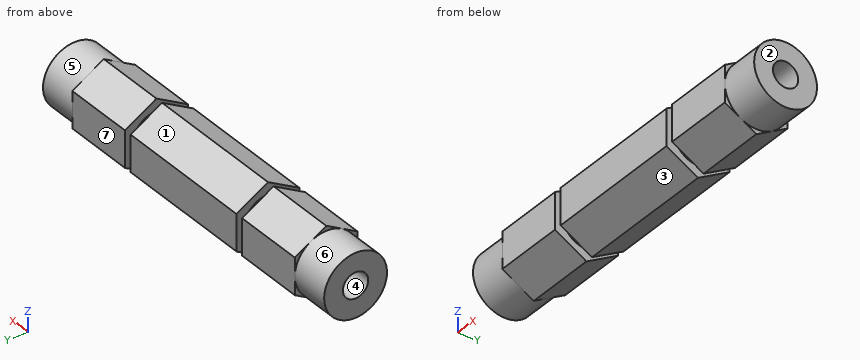
Autodesk Inventor part; units mm, degrees
ref_plane "YZ Plane" through (0, 0, 0) normal (1, 0, 0) x (0, 1, 0)
ref_plane "XZ Plane" through (0, 0, 0) normal (0, 1, 0) x (-1, 0, 0)
ref_plane "XY Plane" through (0, 0, 0) normal (0, 0, 1) x (1, 0, 0)
sketch "Sketch1" plane through (0, 0, 0) normal (1, 0, 0) x (0, 1, 0)
  line L0 (0, -7.3323) -> (-6.35, -3.6662)
  line L1 (-6.35, -3.6662) -> (-6.35, 3.6662)
  line L2 (-6.35, 3.6662) -> (0, 7.3323)
  line L3 (0, 7.3323) -> (6.35, 3.6662)
  line L4 (6.35, 3.6662) -> (6.35, -3.6662)
  line L5 (6.35, -3.6662) -> (0, -7.3323)
  point P0 (0, 0)
  point P1 (0, 0)
  dimension "d0" = 12.7
extrude "Extrusion1" add sketch "Sketch1" along normal mid plane 60.2996
sketch "Sketch2" plane through (-30.1498, 0, 0) normal (-1, 0, 0) x (0, 0, 1)
  circle A0 centre (0, 0) radius 6.35
  dimension "d3" = 12.7
extrude "Extrusion2" add sketch "Sketch2" along normal blind 7.9502
sketch "Sketch3" plane through (30.1498, 0, 0) normal (1, 0, 0) x (0, 0, -1)
  circle A0 centre (0, 0) radius 6.35
  line L0 (3.6662, 6.35) -> (-3.6662, 6.35)
  line L1 (-3.6662, 6.35) -> (-7.3323, 0)
  line L2 (-7.3323, 0) -> (-3.6662, -6.35)
  line L3 (-3.6662, -6.35) -> (3.6662, -6.35)
  line L4 (3.6662, -6.35) -> (7.3323, 0)
  line L5 (7.3323, 0) -> (3.6662, 6.35)
  dimension "d6" = 12.7
extrude "Extrusion3" add sketch "Sketch3" along normal blind 7.9502 contours A0
sketch "Sketch4" plane through (38.1, 0, 0) normal (1, 0, 0) x (0, 0, -1)
  point P0 (0, 0)
  point P1 (0, 0)
hole "Hole1" at (38.1, 0, 0) direction (-1, 0, 0) diameter 5.1054 end through all
sketch "Sketch6" plane through (0, 0, 0) normal (0, 1, 0) x (-1, 0, 0)
  line L0 (30.1498, 6.35) -> (38.1, 6.35)
  line L1 (38.1, 6.35) -> (38.1, 2.5527)
  line L2 (38.1, 2.5527) -> (-38.1, 2.5527)
  line L3 (-38.1, 2.5527) -> (-38.1, 6.35)
  line L4 (-38.1, 6.35) -> (-30.1498, 6.35)
  line L5 (-30.1498, 6.35) -> (-30.1498, 7.3323)
  line L6 (-30.1498, 7.3323) -> (30.1498, 7.3323)
  line L7 (30.1498, 7.3323) -> (30.1498, 6.35)
  line L8 (38.1, -6.35) -> (30.1498, -6.35)
  line L9 (30.1498, -6.35) -> (30.1498, -7.3323)
  line L10 (30.1498, -7.3323) -> (-30.1498, -7.3323)
  line L11 (-30.1498, -7.3323) -> (-30.1498, -6.35)
  line L12 (-30.1498, -6.35) -> (-38.1, -6.35)
  line L13 (-38.1, -6.35) -> (-38.1, -2.5527)
  line L14 (-38.1, -2.5527) -> (38.1, -2.5527)
  line L15 (38.1, -2.5527) -> (38.1, -6.35)
  line L16 (38.1, 2.5527) -> (38.1, -2.5527)
  line L17 (38.1, 0) -> (-38.1, 0)
  line L18 (-38.1, 6.35) -> (-38.1, -6.35)
  line L19 (15.875, -7.3323) -> (14.351, -7.3323)
  line L20 (14.351, -7.3323) -> (14.351, -4.9784)
  line L21 (14.351, -4.9784) -> (15.875, -4.9784)
  line L22 (15.875, -4.9784) -> (15.875, -7.3323)
  point P0 (0, 0)
  dimension "d16" = 9.9568
  dimension "d17" = 1.524
  dimension "d18" = 22.225
revolve "Revolution1" cut sketch "Sketch6" angle 360 about axis through (-38.1, 0, 0) along (1, 0, 0) contours L10 L20 L21 L22
mirror "Mirror1" about plane through (0, 0, 0) normal (1, 0, 0) of "Revolution1"
properties part number "EL2-GB-005E-grove" material "Aluminum 6061"
Design review of the part built by this model. Coordinates are the model's own, in mm. Face numbers are marked on the shaded views. A direction names the side the tool comes from. Give positions to 0.01 mm unless a question says otherwise; leave off trailing zeros. Write each loop counter-clockwise with the first axis right and the second up, starting at its lowest first coordinate (ties: lowest second). Pieces come first, ordered by that corner, then holes. Notation, with made-up numbers: (27, 86) -> (31, 86) arc R15 ccw to (31, 110) -> close; hole circle Ø10 at (-23, -13). An arc over 180 degrees is marked (long way). Answer in a Markdown table with one row per item.
(1) To check wall thickness, follow probe 1 along X at (y, z) = (3.5, 4) (3 decimals); probe 2 along X at (y, z) = (0.25, 6.5) (3 decimals); probe 3 along Y at (x, z) = (13, 0.25). State the ranges of each line that lie inside material, in increasing order.
Results:
| item | result |
|---|---|
| probe 1 | -38.1 to -15.875, -14.351 to 14.351, 15.875 to 38.1 |
| probe 2 | -30.15 to -15.875, -14.351 to 14.351, 15.875 to 30.15 |
| probe 3 | -6.35 to -2.54, 2.54 to 6.35 |
(2) Clearance check with flat-ended pins moving along their axes: pin 1 (4.5 mm diameter, centred on y = 0, z = 0, fed in from -X); pin 2 (1 mm diameter, centred on x = -18, y = -2, fed in from +Z); pin 3 (1 mm diameter, centred on x = -29, y = 1, fed in from +Z). State where each tip first meets the part, or that it passes through.
Results:
| item | result |
|---|---|
| pin 1 | through |
| pin 2 | z = 6.47 |
| pin 3 | z = 7.04 |
(3) Consider section A-A (x = 11). State the section outline as (y, z) points.
Results:
| item | result |
|---|---|
| outline | (-6.35, -3.67) -> (0, -7.33) -> (6.35, -3.67) -> (6.35, 3.67) -> (0, 7.33) -> (-6.35, 3.67) -> close; hole circle Ø5.11 at (0, 0) |
(4) Mouldability with a two-part tool opening along Z and no side actions: class the marked faces 1, 2, 3 and 4 as +Z half, -Z half, draft (parallel to the pull), parting line (faces both ways), or undercut.
Results:
| item | result |
|---|---|
| face 1 | +Z half |
| face 2 | draft |
| face 3 | -Z half |
| face 4 | undercut |
(5) For the marked faces 5, 6 and 7, list the 3-axis set-ups (+Z, -Z, +X, -X, +Y, -Y) from which the entire face can be reached by the end or side of a thin tool; tool diameter is ignored.
Results:
| item | result |
|---|---|
| face 5 | +X |
| face 6 | -X |
| face 7 | +Z, -Z, +X, -X, +Y |
(6) Consider section D-D (y = -4.25). State the section outline as (x, z) points (3 decimals), then the cut area to 3 significant figures.
Results:
| item | result |
|---|---|
| outline | (-38.1, -4.718) -> (-30.15, -4.718) -> (-30.15, -4.879) -> (-15.875, -4.879) -> (-15.875, -2.593) -> (-14.351, -2.593) -> (-14.351, -4.879) -> (14.351, -4.879) -> (14.351, -2.593) -> (15.875, -2.593) -> (15.875, -4.879) -> (30.15, -4.879) -> (30.15, -4.718) -> (38.1, -4.718) -> (38.1, 4.718) -> (30.15, 4.718) -> (30.15, 4.879) -> (15.875, 4.879) -> (15.875, 2.593) -> (14.351, 2.593) -> (14.351, 4.879) -> (-14.351, 4.879) -> (-14.351, 2.593) -> (-15.875, 2.593) -> (-15.875, 4.879) -> (-30.15, 4.879) -> (-30.15, 4.718) -> (-38.1, 4.718) -> close |
| area | 724 mm2 |
